Design review of the part shown in the three views and the two pictorial views. Dimensions are in mm from the part's minimum x, y and z. A direction names the side the tool comes from. Round coordinates to 2 decimals unless told otherwise and drop trailing zeros. Loops run counter-clockwise (first coordinate to the right, second up) from the corner with the lowest first, then second, coordinate; pieces in that order, holes last. Notation, with made-up numbers: (38.5, 80) - (97.5, 80) arc R24 cw to (97.5, 109) - close; hole circle Ø3 at (-11.75, 65.25). An arc over 180 degrees is marked (long way). Return JSON: item names as keys, results as strings. Group by question number.
(1) We need section A-A, the plane z = 6. Write out the cut boundary in (x, y) (3 decimals).
(2) Wall thickness on L1, parallel to X at y = 10.25, z = 7.25; L2, parallel to X at y = 1.8, z = 6 (3 decimals); L3, parallel to Y at x = 10.5, z = 5: over which ranges is each line inside the solid? List them lowest first. Write a range as [from, to].
(3) Clearance check with flat-ended pins moving along their axes: pin 1 (4 mm diameter, centred on x = 9.5, y = 5.5, fed in from -Z); pin 2 (2 mm diameter, centred on x = 3.925, z = 6, fed in from -Y); pin 3 (3.5 mm diameter, centred on x = 12, z = 6.5, fed in from +Y). State where each tip first meets the part, or that it passes through.
(4) We need section D-D, the plane x = 12.75. Write out the cut boundary in (y, z).
(5) The part is to be moulded in two halves that separate along Z. For the marked faces 3, 4, 5 and 6, say which applies: pulls with the +Z half, pulls with the -Z half, needs draft (parallel to the pull), parting line crosses it, or undercut.
(6) For the marked faces 1 and 2, list the 3-axis set-ups (+Z, -Z, +X, -X, +Y, -Y) from which the entire face can be reached by the end or side of a thin tool; tool diameter is ignored.
(7) We need section C-C, the plane z = 10.75. Write out the cut boundary in (x, y).
(8) We need section B-B, the plane y = 7.5. Write out the cut boundary in (x, z).
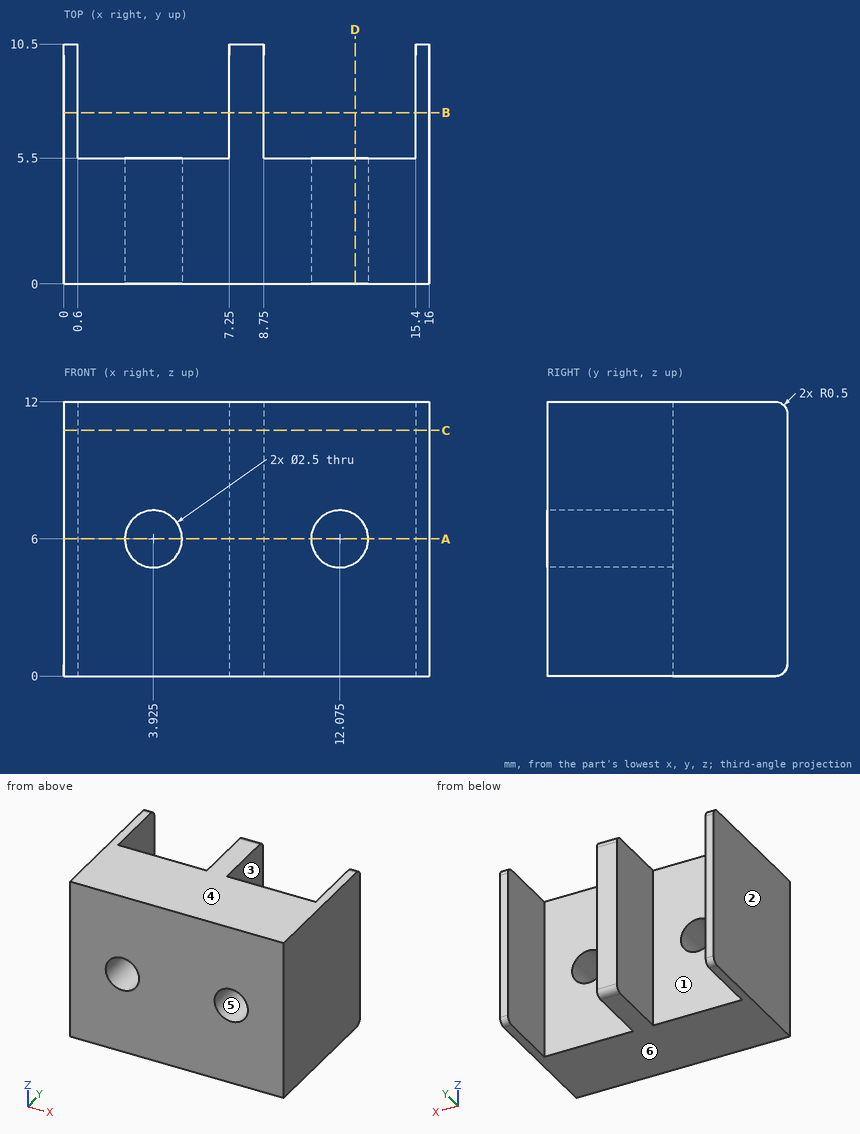
Solutions:
{
 "1": {"outline": "(0, 0) - (2.675, 0) - (2.675, 5.5) - (0.6, 5.5) - (0.6, 10.5) - (0, 10.5) - close; (5.175, 0) - (10.825, 0) - (10.825, 5.5) - (8.75, 5.5) - (8.75, 10.5) - (7.25, 10.5) - (7.25, 5.5) - (5.175, 5.5) - close; (13.325, 0) - (16, 0) - (16, 10.5) - (15.4, 10.5) - (15.4, 5.5) - (13.325, 5.5) - close"},
 "2": {"L1": "[0, 0.6], [7.25, 8.75], [15.4, 16]", "L2": "[0, 2.675], [5.175, 10.825], [13.325, 16]", "L3": "[0, 5.5]"},
 "3": {"pin 1": "z = 0", "pin 2": "through", "pin 3": "y = 5.5"},
 "4": {"outline": "(0, 0) - (5.5, 0) - (5.5, 4.95) - (0, 4.95) - close; (0, 7.05) - (5.5, 7.05) - (5.5, 12) - (0, 12) - close"},
 "5": {"face 3": "needs draft", "face 4": "pulls with the +Z half", "face 5": "undercut", "face 6": "pulls with the -Z half"},
 "6": {"face 1": "+Z, -Z, +Y", "face 2": "+Z, -Z, -X, +Y, -Y"},
 "7": {"outline": "(0, 0) - (16, 0) - (16, 10.5) - (15.4, 10.5) - (15.4, 5.5) - (8.75, 5.5) - (8.75, 10.5) - (7.25, 10.5) - (7.25, 5.5) - (0.6, 5.5) - (0.6, 10.5) - (0, 10.5) - close"},
 "8": {"outline": "(0, 0) - (0.6, 0) - (0.6, 12) - (0, 12) - close; (7.25, 0) - (8.75, 0) - (8.75, 12) - (7.25, 12) - close; (15.4, 0) - (16, 0) - (16, 12) - (15.4, 12) - close"}
}
